Could you check a few things on this model? Use its own coordinates, in mm. A direction names the side the tool comes from. Coordinates: 2 decimals unless noted, no trailing zeros. Loops run counter-clockwise (first coordinate to the right, second up) from the corner with the lowest first, then second, coordinate; pieces in that order, holes last.
1) If I drill on line 1 along X through (y, z) = (249.5, -9); line 2 along Z through (x, y) = (-513, 487.5), over which ranges is the centre line in solid material (lowest first)?
2) Imagine slicing it at B-B on x = -111.5. Please give me the cut outline in (y, z).
3) Will these pins go through, and if not, where does the flat tip stop? P1, Ø5, axis at y = -345.5, z = -0.5, coming from the +X side; P2, Ø8, axis at y = 345.5, z = -34.5, coming from the +X side; P3, Ø12, axis at x = 277, y = -384.5, coming from the -Z side; P4, Ø8, axis at x = -168.5, z = -7, coming from the +Y side.
4) For faces 4 (the face through (-6, 457.2, -25)), 5 (the face through (457.2, -6, -25)), 6 (the face through (-431.8, -6, -25)), which set-ups out of +Z, -Z, +X, -X, +Y, -Y let a thin tool reach every point of the face, with its end or its side?
5) Imagine slicing it at A-A on z = -28.5. Please give me the cut outline in (x, y).
6) Thinking about a two-plate mould opening in Y: for faces 1 (the face through (-6, 431.8, -25)), 2 (the face through (-36, -438, -50.8)), 3 (the face through (-6, -457.2, -25)), which applies, released by +Y, released by -Y, zero draft, split by the parting line, or undercut?
```python
from build123d import *

# Parameters (mm, degrees)
F0_W     = 1219.2
F0_H     = 1219.2
F0_W_2   = 914.4
F0_H_2   = 914.4
F1_DEPTH = 6.35
F2_W     = 914.4
F2_H     = 914.4
F2_W_2   = 863.6
F2_H_2   = 863.6
F3_DEPTH = 57.15


with BuildPart() as f1:
    # F0 (on Top) → F1 (new body)
    with BuildSketch(Plane.XY):
        Rectangle(F0_W, F0_H)
        Rectangle(F0_W_2, F0_H_2, mode=Mode.SUBTRACT)
        Rectangle(F0_W_2, F0_H_2)
    extrude(amount=F1_DEPTH)

    # F2 (on face) → F3 (join)
    with BuildSketch(Plane.XY.offset(6.35)):
        Rectangle(F2_W, F2_H)
        Rectangle(F2_W_2, F2_H_2, mode=Mode.SUBTRACT)
    extrude(amount=-F3_DEPTH)


solid = f1.part
```
Filled in:
1. line 1: x = -457.2 to -431.8, 431.8 to 457.2
1. line 2: z = 0 to 6.35
2. outline: (-609.6, 0) - (-457.2, 0) - (-457.2, -50.8) - (-431.8, -50.8) - (-431.8, 0) - (431.8, 0) - (431.8, -50.8) - (457.2, -50.8) - (457.2, 0) - (609.6, 0) - (609.6, 6.35) - (-609.6, 6.35) - close
3. P1: stops at x = 609.6
3. P2: stops at x = 457.2
3. P3: stops at z = 0
3. P4: stops at y = 457.2
4. face 4: -Z, +X, -X, +Y
4. face 5: -Z, +X, +Y, -Y
4. face 6: -Z
5. outline: (-457.2, -457.2) - (457.2, -457.2) - (457.2, 457.2) - (-457.2, 457.2) - close; hole (-431.8, -431.8) - (431.8, -431.8) - (431.8, 431.8) - (-431.8, 431.8) - close
6. face 1: undercut
6. face 2: zero draft
6. face 3: released by -Y
